Geometry check sheet. Reference: drawing and pictorial views, mm from the part's lowest x, y, z. Round coordinates to 2 decimals unless told otherwise and drop trailing zeros. Order: outer loops, then holes, each group sorted by start corner. A loop starts at its lowest first (then second) coordinate and runs counter-clockwise, first axis right, second up.
Q1. Cross-section at C-C on z = 5. Record the cut outline in (x, y), then the cut area to 3 significant figures.
Q2. Scan lines: probe 1 along Y at (x, z) = (1.25, 7.5); probe 2 along Z at (x, y) = (1.8, 0.95); probe 3 along Y at (x, z) = (1.85, 8). Record each from-to range of solid material in increasing order.
Q3. Cross-section at D-D on z = 1.25. Record the cut outline in (x, y).
Q4. Cross-section at A-A on x = 1.25. Record the cut outline in (y, z), then the cut area to 3 significant figures.
Q5. Mould release check, pull along Y, two halves, no side actions. Record for the marked faces 1, 2 and 3: +Y half, -Y half, draft (parallel to the pull), parting line (faces both ways), or undercut.
Q6. Depth check by flat-ended pin: P1, Ø1, axis at x = 2, y = 1, coming from the -Z side; P2, Ø1.5, axis at y = 0.5, z = 6.5, coming from the +X side. Enter the tip coordinate at first touch or a pass-through.
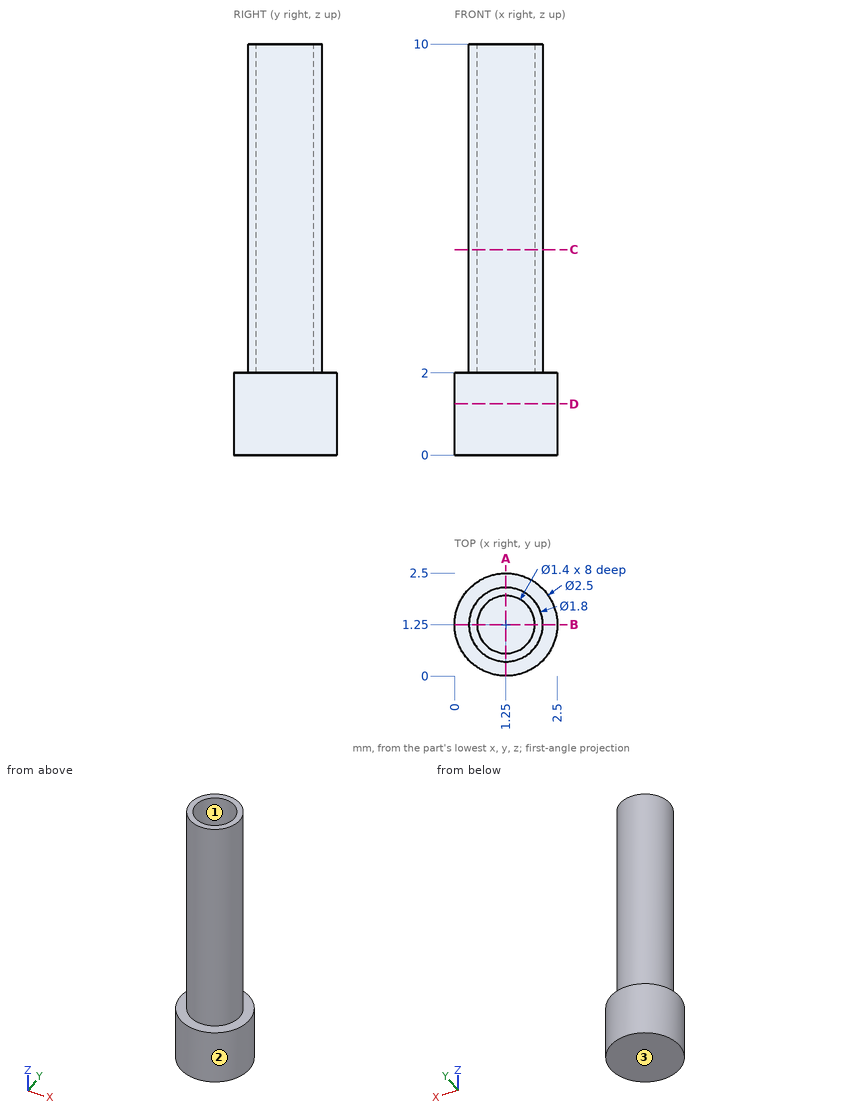
Results found:
1. outline: circle Ø1.8 at (1.25, 1.25); hole circle Ø1.4 at (1.25, 1.25)
1. area: 1.01 mm2
2. probe 1: y = 0.35 to 0.55, 1.95 to 2.15
2. probe 2: z = 0 to 2
2. probe 3: y = 0.58 to 0.89, 1.61 to 1.92
3. outline: circle Ø2.5 at (1.25, 1.25)
4. outline: (0, 0) - (2.5, 0) - (2.5, 2) - (2.15, 2) - (2.15, 10) - (1.95, 10) - (1.95, 2) - (0.55, 2) - (0.55, 10) - (0.35, 10) - (0.35, 2) - (0, 2) - close
4. area: 8.20 mm2
5. face 1: undercut
5. face 2: parting line
5. face 3: draft
6. P1: stops at z = 0
6. P2: stops at x = 2.15
